Geometry: final body of the model. Coordinates: model frame, mm. Round coordinates to 2 decimals unless told otherwise and drop trailing zeros. Loops run counter-clockwise (first coordinate to the right, second up) from the corner with the lowest first, then second, coordinate; pieces in that order, holes last. Notation, with made-up numbers: M -32.5,-16 L 19.5,-16 A27 cw 19.5,2 Z; hole C -1.5,9 d6. An arc over 180 degrees is marked long. Write each question's results on one line, items separated by ' | '.
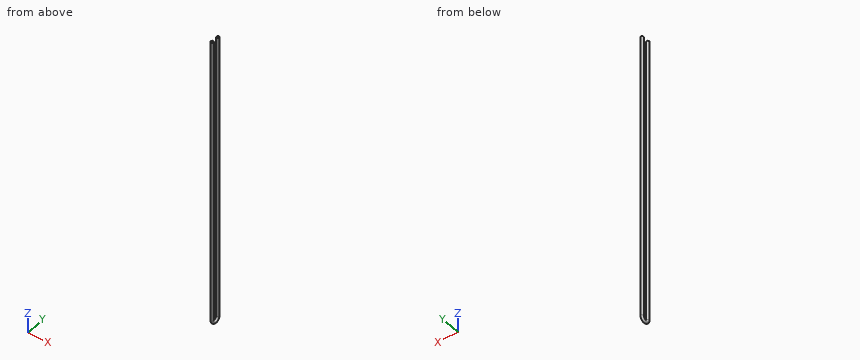
```python
from build123d import *

# Parameters (mm, degrees)
SKETCH2_R   = 10.65
SKETCH2_R_2 = 6.92


with BuildPart() as part:
    # Sweep1: sweep along a path in Sketch1
    with BuildLine(Plane(origin=(0, 0, 0), x_dir=(0, 0, -1), z_dir=(1, 0, 0))) as sweep1_path:
        Line((0, 30), (2325, 30))
        ThreePointArc((2325, 30), (2355, 0), (2325, -30))
        Line((2325, -30), (0, -30))
    # Sketch2 → Sweep1 (sweep)
    with BuildSketch(Plane.XY):
        with Locations((0, 30)):
            Circle(SKETCH2_R)
        with Locations((0, 30)):
            Circle(SKETCH2_R_2, mode=Mode.SUBTRACT)
    sweep(path=sweep1_path.line)


solid = part.part
```
1. Pin query (flat end, axial travel): P1, Ø2, axis at x = 5.5, y = 6, coming from the +Z side; P2, Ø1.5, axis at x = -6.5, y = -10, coming from the +Z side; P3, Ø2, axis at y = 25.5, z = -578, coming from the +X side. Return the tip coordinate at first contact, or that it passes through.
Answer key:
P1: stops at z = -2344.35 | P2: stops at z = -2343.37 | P3: stops at x = 10.06
2. Section A-A (x = 1). Output: boundary loops of the cut face in (y, z), then the cut area to 3 significant figures.
Answer key:
outline: M -40.6,-2325 A40.6 ccw 40.6,-2325 L 40.6,0 L 36.85,0 L 36.85,-2325 A36.85 cw -36.85,-2325 L -36.85,0 L -40.6,0 Z; M -23.15,-2325 A23.15 ccw 23.15,-2325 L 23.15,0 L 19.4,0 L 19.4,-2325 A19.4 cw -19.4,-2325 L -19.4,0 L -23.15,0 Z | area: 35,600 mm²
3. Section B-B (z = -313). Output: boundary loops of the cut face in (x, y).
Answer key:
outline: C 0,-30 d21.3; C 0,30 d21.3; hole C 0,-30 d13.84; hole C 0,30 d13.84
4. Ray query, probe 1 along Y at (x, z) = (-2.5, -376); probe 2 along Y at (x, z) = (0.75, -574); probe 3 along X at (y, z) = (-30.5, -2151). Return the intervals inside material, ascending.
Answer key:
probe 1: y = -40.35 to -36.45, -23.55 to -19.65, 19.65 to 23.55, 36.45 to 40.35 | probe 2: y = -40.62 to -36.88, -23.12 to -19.38, 19.38 to 23.12, 36.88 to 40.62 | probe 3: x = -10.64 to -6.9, 6.9 to 10.64
